The listing builds one solid part. Answer for the finished solid, in the listing's coordinates (mm). A direction names the side the tool comes from. Coordinates: 2 decimals unless noted, no trailing zeros. Write each loop counter-clockwise with the first axis right and the second up, starting at its lowest first coordinate (ties: lowest second). Pieces come first, ordered by that corner, then holes. Notation, with made-up numbers: M -3,23.25 L 39,23.25 A9 cw 39,33.25 Z; hole C 47,-38 d6. An arc over 180 degrees is marked long. Answer as a JSON object with one key per item and string values. Group by question number.
from build123d import *

# Parameters (mm, degrees)
SKETCH2_R             = 32.5
SKETCH2_R_2           = 6.5
SKETCH2_R_3           = 1.5
BOSS_EXTRUDE1_DEPTH   = 10
M5X0_8_TAPPED_HOLE1_D = 4.2
BOSS_EXTRUDE2_START   = -6.5
SKETCH8_R             = 6.5
BOSS_EXTRUDE2_DEPTH   = 6.5
SKETCH9_R             = 32.5
SKETCH9_R_2           = 17.5
CUT_EXTRUDE1_DEPTH    = 1
SKETCH10_W            = 1.5
SKETCH10_H            = 2
M5X0_8_TAPPED_HOLE2_D = 4.2


with BuildPart() as part:
    # Sketch2 → Boss-Extrude1 (new body)
    with BuildSketch(Plane(origin=(0, 0, 0), x_dir=(1, 0, 0), z_dir=(0, 1, 0))):
        with Locations(Location((0, 0, 0), (0, 0, 270))):
            Circle(SKETCH2_R)
        with Locations(Location((0, 0, 0), (0, 0, 270))):
            Circle(SKETCH2_R_2, mode=Mode.SUBTRACT)
        with Locations(Location((27.25, 0, 0), (0, 0, 270))):
            Circle(SKETCH2_R_3, mode=Mode.SUBTRACT)
        with Locations(Location((13.625, -23.599192253, 0), (0, 0, 270))):
            Circle(SKETCH2_R_3, mode=Mode.SUBTRACT)
        with Locations(Location((-13.625, -23.599192253, 0), (0, 0, 270))):
            Circle(SKETCH2_R_3, mode=Mode.SUBTRACT)
        with Locations(Location((-27.25, 0, 0), (0, 0, 270))):
            Circle(SKETCH2_R_3, mode=Mode.SUBTRACT)
        with Locations(Location((-13.625, 23.599192253, 0), (0, 0, 270))):
            Circle(SKETCH2_R_3, mode=Mode.SUBTRACT)
        with Locations(Location((13.625, 23.599192253, 0), (0, 0, 270))):
            Circle(SKETCH2_R_3, mode=Mode.SUBTRACT)
    extrude(amount=BOSS_EXTRUDE1_DEPTH)

    # M5x0.8 Tapped Hole1 (through all)
    with Locations(Plane(origin=(0, 10, 0), x_dir=(1, 0, 0), z_dir=(0, 1, 0))):
        with Locations((-13.625, 23.599192253), (13.625, 23.599192253), (27.25, 0), (13.625, -23.599192253), (-13.625, -23.599192253), (-27.25, 0)):
            Hole(M5X0_8_TAPPED_HOLE1_D / 2)

    # Sketch8 → Boss-Extrude2 (add)
    with BuildSketch(Plane(origin=(0, 10, 0), x_dir=(1, 0, 0), z_dir=(0, 1, 0)).offset(BOSS_EXTRUDE2_START)):
        with Locations(Location((0, 0, 0), (0, 0, 270))):
            Circle(SKETCH8_R)
    extrude(amount=BOSS_EXTRUDE2_DEPTH)

    # Sketch9 → Cut-Extrude1 (cut)
    with BuildSketch(Plane.XZ):
        with Locations(Location((0, 0, 0), (0, 0, 270))):
            Circle(SKETCH9_R)
        with Locations(Location((0, 0, 0), (0, 0, 270))):
            Circle(SKETCH9_R_2, mode=Mode.SUBTRACT)
    extrude(amount=-CUT_EXTRUDE1_DEPTH, mode=Mode.SUBTRACT)

    # Sketch10 → Revolve1 (revolve)
    with BuildSketch(Plane(origin=(0, 0, 0), x_dir=(0, 0, -1), z_dir=(1, 0, 0)), mode=Mode.PRIVATE) as revolve1_sk:
        with Locations((-33.25, 2)):
            Rectangle(SKETCH10_W, SKETCH10_H)
    revolve(revolve1_sk.sketch.rotate(Axis((0, 0, 0), (0, 1, 0)), 180), axis=Axis((0, 0, 0), (0, 1, 0)))

    # M5x0.8 Tapped Hole2 (through all)
    with Locations(Plane(origin=(0, 10, 0), x_dir=(1, 0, 0), z_dir=(0, 1, 0))):
        with Locations((0, 22.5), (19.485571585, 11.25), (19.485571585, -11.25), (0, -22.5), (-19.485571585, -11.25), (-19.485571585, 11.25)):
            Hole(M5X0_8_TAPPED_HOLE2_D / 2)


solid = part.part
Item 1: A tool of negligible diameter and unlimited length cuts with its end or side. For faces 1 (the face through (17, 3, -28)), 2 (the face through (-19.21, 5.44, -13.33)), 3 (the face through (-3.955, 1.726, -5.158)), from which of +Z, -Z, +X, -X, +Y, -Y can it reach the whole face along a straight path? Write none if from no direction.
Item 2: Consider L1, parallel to X at y = 8, z = 22.5; L2, parallel to X at y = 2.5, z = -25; L3, parallel to X at y = 6.5, z = -11.25. Determine where each line is inside the solid, lowest interval first. Write a range as from..to.
Item 3: For a pull along X with two mould halves and no side action, classify faces 4 (the face through (-16, 1, 8)), 5 (the face through (-14.754, 5.437, 21.828)), 6 (the face through (-10.648, 0.493, 13.887)) as +X half, -X half, draft (parallel to the pull), parting line (faces both ways), or undercut.
Item 4: A cutting plane is placed at A-A, the plane x = 0. Write down the section's boundary in (y, z), and give its area (3 significant figures).
Item 5: A cutting plane is placed at D-D, the plane z = -22.5. Write down the section's boundary in (x, y), and give its area (3 significant figures).
Item 6: A cutting plane is placed at B-B, the plane z = 12.5. Write down the section's boundary in (x, y), and give its area (3 significant figures).
Item 7: Flat-ended cylindrical pins translate along their axes: pin 1 Ø2 at (y, z) = (1.5, -17.5) entering from +X; pin 2 Ø4 at (x, z) = (-19.49, 11.25) entering from -Y; pin 3 Ø10.5 at (x, z) = (0, 0) entering from -Y; pin 4 Ø6.5 at (x, z) = (-13.62, -23.6) entering from -Y. Find the tip coordinate at first contact, or state that the pin passes through.
Item 8: A cutting plane is placed at C-C, the plane x = -28.5. Write down the section's boundary in (y, z).
Answer:
{
 "1": {"face 1": "+Y", "face 2": "+Y, -Y", "face 3": "-Y"},
 "2": {"L1": "-23.45..-15.41, -11.84..-2.1, 2.1..11.84, 15.41..23.45", "L2": "-23.04..-15.19, -12.06..12.06, 15.19..23.04", "L3": "-30.49..-21.59, -17.39..17.39, 21.59..30.49"},
 "3": {"face 4": "draft", "face 5": "undercut", "face 6": "parting line"},
 "4": {"outline": "M 0,-17.5 L 1,-17.5 L 1,-20.4 L 10,-20.4 L 10,20.4 L 1,20.4 L 1,17.5 L 0,17.5 L 0,6.5 L 3.5,6.5 L 3.5,-6.5 L 0,-6.5 Z; M 1,-34 L 3,-34 L 3,-32.5 L 10,-32.5 L 10,-24.6 L 1,-24.6 Z; M 1,24.6 L 10,24.6 L 10,32.5 L 3,32.5 L 3,34 L 1,34 Z", "area": "505 mm2"},
 "5": {"outline": "M -25.49,1 L -15.41,1 L -15.41,10 L -23.45,10 L -23.45,3 L -25.49,3 Z; M -11.84,1 L -2.1,1 L -2.1,10 L -11.84,10 Z; M 2.1,1 L 11.84,1 L 11.84,10 L 2.1,10 Z; M 15.41,1 L 25.49,1 L 25.49,3 L 23.45,3 L 23.45,10 L 15.41,10 Z", "area": "328 mm2"},
 "6": {"outline": "M -31.62,1 L -21.17,1 L -21.17,10 L -30,10 L -30,3 L -31.62,3 Z; M -17.8,1 L -12.25,1 L -12.25,0 L 12.25,0 L 12.25,1 L 17.8,1 L 17.8,10 L -17.8,10 Z; M 21.17,1 L 31.62,1 L 31.62,3 L 30,3 L 30,10 L 21.17,10 Z", "area": "510 mm2"},
 "7": {"pin 1": "x = 29.73", "pin 2": "through", "pin 3": "y = 3.5", "pin 4": "y = 1"},
 "8": {"outline": "M 1,-18.54 L 3,-18.54 L 3,-15.62 L 10,-15.62 L 10,-1.69 L 1,-1.69 Z; M 1,1.69 L 10,1.69 L 10,15.62 L 3,15.62 L 3,18.54 L 1,18.54 Z"}
}
